Input: part model. Units: mm. Frame: model coordinates. Round coordinates to 2 decimals unless told otherwise and drop trailing zeros. Loops run counter-clockwise (first coordinate to the right, second up) from the corner with the lowest first, then second, coordinate; pieces in that order, holes last. Notation, with made-up numbers: M 60.25,13 L 64.25,13 A23 cw 64.25,36 Z; hole C 3,17 d10. An arc over 180 degrees is marked long. Return JSON: item names as keys, results as strings. Group by question number.
1) Contact query for flat-ended pins moving along their axis: P1, Ø4, axis at x = 0, y = 1, coming from the -Z side; P2, Ø4, axis at x = -1, z = 22, coming from the -Y side; P3, Ø5, axis at y = -3, z = 11.5, coming from the -X side; P4, Ø1.5, axis at x = 3, y = 4.5, coming from the +Z side. Output: stop coordinate, or through.
2) Section C-C (z = 4.25). Output: boundary loops of the cut face in (x, y), plus the area to 3 significant figures.
3) Section A-A (x = 0). Output: boundary loops of the cut face in (y, z), plus the area to 3 significant figures.
4) Material intervals for line 1 (Y direction, x = 0.25, z = 9); line 2 (Z direction, x = 0.75, y = 3.5); line 3 (Y direction, x = 2.75, z = 21), sorted ascending. Write a range as from..to.
from build123d import *

# Parameters (mm, degrees)
F0_R     = 6
F1_DEPTH = 25
F2_R     = 6
F3_SIZE2 = 1.732051
F3_SIZE  = 3


with BuildPart() as f1:
    # F0 (on Top) → F1 (new body)
    with BuildSketch(Plane.XY):
        Circle(F0_R)
    extrude(amount=F1_DEPTH)

    # F2
    f2_edges = [f1.edges().sort_by_distance(p)[0] for p in [
        (-6, 0, 25),
    ]]
    fillet(f2_edges, radius=F2_R)

    # F3
    f3_edges = [f1.edges().sort_by_distance(p)[0] for p in [
        (-6, 0, 0),
    ]]
    chamfer(f3_edges, length=F3_SIZE, length2=F3_SIZE2)


solid = f1.part
Returned:
{
 "1": {"P1": "stops at z = 0", "P2": "stops at y = -5.89", "P3": "stops at x = -5.98", "P4": "stops at z = 22.78"},
 "2": {"outline": "C 0,0 d12", "area": "113 mm^2"},
 "3": {"outline": "M -6,3 L -4.27,0 L 4.27,0 L 6,3 L 6,19 A6 ccw -6,19 Z", "area": "279 mm^2"},
 "4": {"line 1": "y = -5.99..5.99", "line 2": "z = 0..23.82", "line 3": "y = -4.94..4.94"}
}
